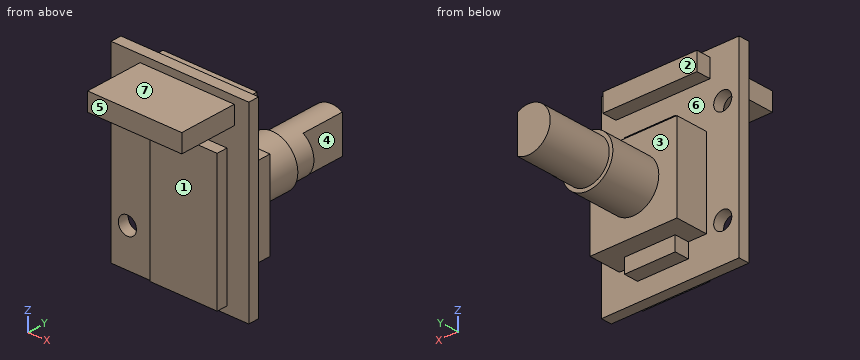
```python
from build123d import *

# Parameters (mm, degrees)
SCHIZZO1_W                        = 19
SCHIZZO1_H                        = 26
ESTRUSIONE_ESTRUSIONE1_DEPTH      = 1.5
SCHIZZO2_W                        = 12
SCHIZZO2_H                        = 12
ESTRUSIONE_ESTRUSIONE2_DEPTH      = 4.5
SCHIZZO4_R                        = 3.5
ESTRUSIONE_ESTRUSIONE3_DEPTH      = 7
SCHIZZO5_R                        = 3
ESTRUSIONE_ESTRUSIONE4_DEPTH      = 9
TAGLIO_ESTRUSIONE1_DEPTH          = 6
SCHIZZO7_R                        = 1.25
TAGLIO_ESTRUSIONE2_DEPTH          = 6
ESTRUSIONE_ESTRUSIONE5_DEPTH      = 2
ESTRUSIONE_ESTRUSIONE5_DEPTH_BACK = 9.5
SCHIZZO8_W                        = 13
SCHIZZO8_H                        = 2.5
SCHIZZO9_W                        = 9.25
SCHIZZO9_H                        = 18.5
ESTRUSIONE_ESTRUSIONE6_DEPTH      = 1.5
SCHIZZO10_W                       = 7
SCHIZZO10_H                       = 2
ESTRUSIONE_ESTRUSIONE7_DEPTH      = 2


with BuildPart() as part:
    # Schizzo1 → Estrusione-Estrusione1 (new body)
    with BuildSketch(Plane(origin=(0, 0, 0), x_dir=(1, 0, 0), z_dir=(0, 1, 0))):
        Rectangle(SCHIZZO1_W, SCHIZZO1_H)
    extrude(amount=ESTRUSIONE_ESTRUSIONE1_DEPTH)

    # Schizzo2 → Estrusione-Estrusione2 (add)
    with BuildSketch(Plane(origin=(0, 1.5, 0), x_dir=(1, 0, 0), z_dir=(0, 1, 0))):
        with Locations((1, 2.5)):
            Rectangle(SCHIZZO2_W, SCHIZZO2_H)
    extrude(amount=ESTRUSIONE_ESTRUSIONE2_DEPTH)

    # Schizzo4 → Estrusione-Estrusione3 (add)
    with BuildSketch(Plane(origin=(0, 6, 0), x_dir=(1, 0, 0), z_dir=(0, 1, 0))):
        with Locations(Location((1, 2.5, 0), (0, 0, 270))):
            Circle(SCHIZZO4_R)
    extrude(amount=ESTRUSIONE_ESTRUSIONE3_DEPTH)

    # Schizzo5 → Estrusione-Estrusione4 (add)
    with BuildSketch(Plane(origin=(0, 13, 0), x_dir=(1, 0, 0), z_dir=(0, 1, 0))):
        with Locations(Location((1, 2.5, 0), (0, 0, 270))):
            Circle(SCHIZZO5_R)
    extrude(amount=ESTRUSIONE_ESTRUSIONE4_DEPTH)

    # Schizzo6 → Taglio-Estrusione1 (cut)
    with BuildSketch(Plane(origin=(0, 22, 0), x_dir=(1, 0, 0), z_dir=(0, 1, 0))):
        Polygon((2.5, 58.528036495), (2.5, 5.098076211), (2.5, -0.098076211), (2.5, -53.528036495), (109.359920567, -53.528036495), (109.359920567, 58.528036495), align=None)
    extrude(amount=-TAGLIO_ESTRUSIONE1_DEPTH, mode=Mode.SUBTRACT)

    # Schizzo7 → Taglio-Estrusione2 (cut)
    with BuildSketch(Plane(origin=(0, 1.5, 0), x_dir=(1, 0, 0), z_dir=(0, 1, 0))):
        with Locations(Location((-7.25, 7.75, 0), (0, 0, 270))):
            Circle(SCHIZZO7_R)
        with Locations(Location((-7.25, -6.25, 0), (0, 0, 270))):
            Circle(SCHIZZO7_R)
    extrude(amount=-TAGLIO_ESTRUSIONE2_DEPTH, mode=Mode.SUBTRACT)

    # Schizzo8 → Estrusione-Estrusione5 (add, two sides: drawn at the far end of the back side and taken through both)
    with BuildSketch(Plane(origin=(0, 1.5, 0), x_dir=(1, 0, 0), z_dir=(0, 1, 0)).offset(-ESTRUSIONE_ESTRUSIONE5_DEPTH_BACK)):
        with Locations((1, -10.75)):
            Rectangle(SCHIZZO8_W, SCHIZZO8_H)
    extrude(amount=ESTRUSIONE_ESTRUSIONE5_DEPTH + ESTRUSIONE_ESTRUSIONE5_DEPTH_BACK)

    # Schizzo9 → Estrusione-Estrusione6 (add)
    with BuildSketch(Plane.XZ):
        with Locations((1.875, -2.75)):
            Rectangle(SCHIZZO9_W, SCHIZZO9_H)
    extrude(amount=ESTRUSIONE_ESTRUSIONE6_DEPTH)

    # Schizzo10 → Estrusione-Estrusione7 (add)
    with BuildSketch(Plane(origin=(0, 1.5, 0), x_dir=(1, 0, 0), z_dir=(0, 1, 0))):
        with Locations((1, 9.5)):
            Rectangle(SCHIZZO10_W, SCHIZZO10_H)
        with Locations((1, -4.5)):
            Rectangle(SCHIZZO10_W, SCHIZZO10_H)
    extrude(amount=ESTRUSIONE_ESTRUSIONE7_DEPTH)


solid = part.part
```
Read the model definition and answer for the solid it produces. Units are mm, in the model's axes. Face numbers are marked on the shaded views. A direction names the side the tool comes from. Give positions to 0.01 mm unless a question says otherwise; leave off trailing zeros. Loops run counter-clockwise (first coordinate to the right, second up) from the corner with the lowest first, then second, coordinate; pieces in that order, holes last.
Item 1: Each of these flat-tipped pins is pushed along its axis until it touches: pin 1 Ø2 at (y, z) = (3.5, -1) entering from -X; pin 2 Ø6 at (x, y) = (-3, 14.5) entering from -Z; pin 3 Ø1 at (x, y) = (2, 2.5) entering from -Z. Where does it stop, or does it pass through?
Item 2: The part is cut by section B-B (z = -7.75). Write down the section's boundary in (x, y).
Item 3: The mould has two halves that part along Z. Classify the marked faces 5, 6 and 7: released by +Z, released by -Z, zero draft, split by the parting line, or undercut.
Item 4: For the marked faces 1, 2, 3 and 4, determine the directions among +Z, -Z, +X, -X, +Y, -Y from which every point of the face is accessible in a straight line to the end or side of a thin tool.
Item 5: Find the intervals of material crossed by line 1 along X through (y, z) = (0.6, 6.25); line 2 along Z through (x, y) = (3.75, -1.25); line 3 along Y through (x, z) = (-5.5, -5.25), in increasing order.
Item 6: The part is cut by section C-C (y = 2.5). Write down the section's boundary in (x, z), and give its area (4 significant figures).
Item 7: The part is cut by section A-A (x = -7.25). Write down the section's boundary in (y, z).
Item 8: The part is cut by section D-D (z = 4.25). Write down the section's boundary in (x, y).
Taken from the geometry:
1. pin 1: stops at x = -5
1. pin 2: stops at z = -5.71
1. pin 3: stops at z = -10.5
2. outline: (-9.5, 0) - (-8.5, 0) - (-8.5, 1.5) - (-9.5, 1.5) - close; (-6, 0) - (-2.75, 0) - (-2.75, -1.5) - (6.5, -1.5) - (6.5, 0) - (9.5, 0) - (9.5, 1.5) - (7, 1.5) - (7, 6) - (-5, 6) - (-5, 1.5) - (-6, 1.5) - close
3. face 5: zero draft
3. face 6: undercut
3. face 7: released by +Z
4. face 1: -Z, +X, -X, -Y
4. face 2: +Z, +X, -X, +Y
4. face 3: +Y
4. face 4: +Z, -Z, +X, +Y
5. line 1: x = -9.5 to -8.5, -6 to 9.5
5. line 2: z = -12 to 6.5, 9.5 to 12
5. line 3: y = 0 to 1.5
6. outline: (-5.5, 9.5) - (7.5, 9.5) - (7.5, 12) - (-5.5, 12) - close; (-5, -8.5) - (-2.5, -8.5) - (-2.5, -10.5) - (4.5, -10.5) - (4.5, -8.5) - (7, -8.5) - (7, 3.5) - (4.5, 3.5) - (4.5, 5.5) - (-2.5, 5.5) - (-2.5, 3.5) - (-5, 3.5) - close
6. area: 204.5 mm2
7. outline: (0, -13) - (1.5, -13) - (1.5, -9) - (0, -9) - close; (0, -6.5) - (1.5, -6.5) - (1.5, 5) - (0, 5) - close; (0, 7.5) - (1.5, 7.5) - (1.5, 13) - (0, 13) - close
8. outline: (-9.5, 0) - (-2.75, 0) - (-2.75, -1.5) - (6.5, -1.5) - (6.5, 0) - (9.5, 0) - (9.5, 1.5) - (4.5, 1.5) - (4.5, 3.5) - (-2.5, 3.5) - (-2.5, 1.5) - (-9.5, 1.5) - close
